from build123d import *

# Parameters (mm, degrees)
F0_W      = 11.55
F0_H      = 1.48
F0_H_2    = 11.79
F1_DEPTH  = 11.33
F2_W      = 11.55
F2_H      = 11.79
F3_DEPTH  = 9.73
F4_W      = 3
F4_H      = 6
F5_DEPTH  = 8
F6_W      = 3
F6_H      = 6
F7_DEPTH  = 8
F8_R      = 4
F9_R      = 3.99999
F10_R     = 4
F11_R     = 3.99999
F12_R     = 1.5
F13_DEPTH = 25
F14_R     = 1.5
F15_DEPTH = 25
F16_SIZE  = 1
F17_SIZE  = 1


# Not quite as in the source:
# - a fillet or chamfer is up to 0.001 mm smaller than in the source, because OpenCascade refuses the exact size


with BuildPart() as f1:
    # F0 (on Front) → F1 (new body)
    with BuildSketch(Plane.XZ):
        with Locations((5.775, 0.74)):
            Rectangle(F0_W, F0_H)
        with Locations((5.775, 14.01)):
            Rectangle(F0_W, F0_H)
        with Locations((5.775, 7.375)):
            Rectangle(F0_W, F0_H_2)
    extrude(amount=F1_DEPTH)

    # F2 (on face) → F3 (cut)
    with BuildSketch(Plane.XZ.offset(11.33)):
        with Locations((5.775, 7.375)):
            Rectangle(F2_W, F2_H)
    extrude(amount=-F3_DEPTH, mode=Mode.SUBTRACT)

    # F4 (on face) → F5 (join)
    with BuildSketch(Plane.YZ.offset(11.55)):
        with Locations((-9.83, 17.75)):
            Rectangle(F4_W, F4_H)
        Polygon((-8.33, 14.75), (-11.33, 14.75), (-11.33, 13.27), (-1.6, 13.27), (-1.6, 1.48), (-11.33, 1.48), (-11.33, 0), (0, 0), (0, 14.75), align=None)
    extrude(amount=-F5_DEPTH)

    # F6 (on face) → F7 (join)
    with BuildSketch(Plane.YZ.offset(11.55)):
        with Locations((-9.83, -3)):
            Rectangle(F6_W, F6_H)
    extrude(amount=-F7_DEPTH)

    # F8
    f8_edges = [f1.edges().sort_by_distance(p)[0] for p in [
        (11.55, -9.83, 20.75),
    ]]
    fillet(f8_edges, radius=F8_R)

    # F9 (radius 4 in the source; OpenCascade refuses exactly that, so slightly less here)
    f9_edges = [f1.edges().sort_by_distance(p)[0] for p in [
        (3.55, -9.83, 20.75),
    ]]
    fillet(f9_edges, radius=F9_R)

    # F10
    f10_edges = [f1.edges().sort_by_distance(p)[0] for p in [
        (11.55, -9.83, -6),
    ]]
    fillet(f10_edges, radius=F10_R)

    # F11 (radius 4 in the source; OpenCascade refuses exactly that, so slightly less here)
    f11_edges = [f1.edges().sort_by_distance(p)[0] for p in [
        (3.55, -9.83, -6),
    ]]
    fillet(f11_edges, radius=F11_R)

    # F12 (on face) → F13 (cut)
    with BuildSketch(Plane(origin=(0, -8.33, 0), x_dir=(-1, 0, 0), z_dir=(0, 1, 0))):
        with Locations((-7.6327412389, -2.4092334788)):
            Circle(F12_R)
    extrude(amount=-F13_DEPTH, mode=Mode.SUBTRACT)

    # F14 (on face) → F15 (cut)
    with BuildSketch(Plane(origin=(0, -8.33, 0), x_dir=(-1, 0, 0), z_dir=(0, 1, 0))):
        with Locations((-7.6965787448, 17.3904672265)):
            Circle(F14_R)
    extrude(amount=-F15_DEPTH, mode=Mode.SUBTRACT)

    # F16
    f16_edges = [f1.edges().sort_by_distance(p)[0] for p in [
        (5.775, -1.6, 13.27),
    ]]
    chamfer(f16_edges, length=F16_SIZE)

    # F17
    f17_edges = [f1.edges().sort_by_distance(p)[0] for p in [
        (5.775, -1.6, 1.48),
    ]]
    chamfer(f17_edges, length=F17_SIZE)


solid = f1.part
Verification items for the finished model (mm, model axes). A direction names the side the tool comes from. Coordinates: 2 decimals unless noted, no trailing zeros. Write each loop counter-clockwise with the first axis right and the second up, starting at its lowest first coordinate (ties: lowest second). Pieces come first, ordered by that corner, then holes. Notation, with made-up numbers: (82.25, 79) -> (123.25, 79) arc R13 cw to (123.25, 101) -> close; hole circle Ø2 at (-36.75, 52.25). An arc over 180 degrees is marked (long way). One line per item, written item: value. Start each with the question number.
Q1. Go/stop test with flat-tipped pins: P1, Ø6, axis at x = 5.5, z = 16, coming from the +Y side; P2, Ø5.5, axis at x = 3.5, y = -8, coming from the -Z side; P3, Ø5, axis at x = 7.5, y = -2, coming from the -Z side; P4, Ø3, axis at x = 2.5, z = 4.5, coming from the -Y side. Record where each tip stops, or that it passes through.
Q2. Cross-section at C-C on y = -9. State how many separate pieces and enclosed holes the cut face has, and give its area (3 significant figures).
Q3. Cross-section at A-A on y = -7. Enter the section's corners in (x, z).
Q4. Cross-section at B-B on x = 1. Enter the section's corners in (y, z).
Q5. Cross-section at D-D on x = 6.5. Enter the section's corners in (y, z).
Q6. Access from +Z, -Z, +X, -X, +Y, -Y to the whole of each face (thin tool, end or side, straight path). Record for faces 1 (the flat face through (7, -8.33, -4)), 2 (the flat face through (5.69, -2.11, 12.78)), 3 (the flat face through (3.55, -10, 16)).
Q7. Mould release check, pull along Z, two halves, no side actions. Record for faces 4 (the flat face through (6, -7, 13.27)), 5 (the cylindrical face through (10.409, -9.809, -4.797)), 6 (the cylindrical face through (4.753, -9.809, 19.609)): pulls with the +Z half, pulls with the -Z half, needs draft (parallel to the pull), parting line crosses it, or undercut.
Q8. Thickness scan on L1, parallel to Z at x = 7.75, y = -9.75 (3 decimals); L2, parallel to Z at x = 6, y = -5.75; L3, parallel to Y at x = 3.75, z = 15.75. Record the ranges inside material, lowest first. Write a range as from..to.
Checked values:
1. P1: stops at y = 0
1. P2: stops at z = -5.78
1. P3: stops at z = 0
1. P4: stops at y = -1.6
2. separate pieces: 2
2. enclosed holes: 2
2. area: 102 mm²
3. outline: (0, 0) -> (11.55, 0) -> (11.55, 1.48) -> (0, 1.48) -> close; (0, 13.27) -> (11.55, 13.27) -> (11.55, 14.75) -> (0, 14.75) -> close
4. outline: (-11.33, 0) -> (0, 0) -> (0, 14.75) -> (-11.33, 14.75) -> (-11.33, 13.27) -> (-2.6, 13.27) -> (-1.6, 12.27) -> (-1.6, 2.48) -> (-2.6, 1.48) -> (-11.33, 1.48) -> close
5. outline: (-11.33, -5.86) -> (-8.33, -5.86) -> (-8.33, -3.39) -> (-11.33, -3.39) -> close; (-11.33, -1.43) -> (-8.33, -1.43) -> (-8.33, 0) -> (0, 0) -> (0, 14.75) -> (-8.33, 14.75) -> (-8.33, 16.49) -> (-11.33, 16.49) -> (-11.33, 13.27) -> (-2.6, 13.27) -> (-1.6, 12.27) -> (-1.6, 2.48) -> (-2.6, 1.48) -> (-11.33, 1.48) -> close; (-11.33, 18.3) -> (-8.33, 18.3) -> (-8.33, 20.61) -> (-11.33, 20.61) -> close
6. face 1: -Z, +X, -X, +Y
6. face 2: +X, -X, -Y
6. face 3: +Z, -X, +Y, -Y
7. face 4: undercut
7. face 5: pulls with the -Z half
7. face 6: pulls with the +Z half
8. L1: z = -5.995..-3.905, -0.914..1.48, 13.27..15.891, 18.89..20.745
8. L2: z = 0..1.48, 13.27..14.75
8. L3: y = -11.33..-8.33
